Input: dimensioned drawing with shaded views. Units: mm. Origin: part minimum x, y, z. A direction names the side the tool comes from. Give positions to 0.01 mm unless a question says otherwise; leave off trailing zeros. Loops run counter-clockwise (first coordinate to the right, second up) from the corner with the lowest first, then second, coordinate; pieces in that order, holes last. Notation, with made-up numbers: (3.25, -5) -> (9.25, -5) arc R6 ccw to (9.25, 5) -> close; hole circle Ø11 at (65.25, 51). An arc over 180 degrees is marked (long way). One line per question, with ' | ' between items. Start each with the question number.
Item 1: Set-up query: the marked faces 4, 5, 6 and 7. Return all of +Z, -Z, +X, -X, +Y, -Y with unobstructed straight access to the full face (end or side cutting, diameter ignored); none if empty.
Item 2: Pin query (flat end, axial travel): P1, Ø1.9, axis at y = 2, z = 13, coming from the +X side; P2, Ø3, axis at x = 18.5, y = 3.5, coming from the -Z side; P3, Ø1.9, axis at y = 3.5, z = 4, coming from the +X side. Return the tip coordinate at first contact, or that it passes through.
Item 3: Section C-C on z = 24. Return loops of the section in (x, y), then the cut area to 3 significant figures.
Item 4: Section B-B on x = 27.5. Return loops of the section in (y, z).
Item 5: Material intervals for line 1 along X through (y, z) = (2.25, 6); line 2 along X through (y, z) = (1.5, 28.5); line 3 along Z through (x, y) = (10.5, 3.5), sorted ascending. Write a range as [from, to].
Item 6: Mould query, pull axis X, two halves, no side actions, for the marked faces 1, 2 and 3. Classes: released by +X, released by -X, zero draft, split by the parting line, or undercut.
Item 7: Section A-A on y = 4.25. Return loops of the section in (x, z) (3 decimals).
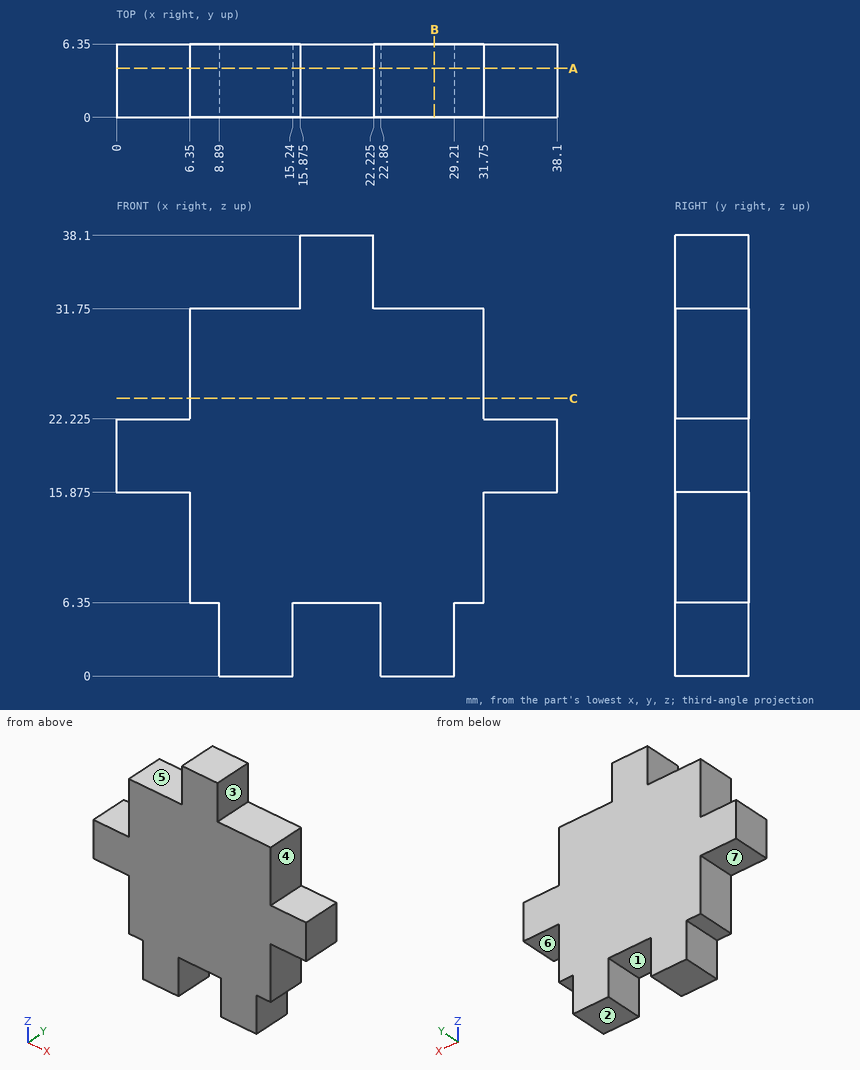
Result sheet:
1) face 4: +Z, +X, +Y, -Y | face 5: +Z, -X, +Y, -Y | face 6: -Z, +X, +Y, -Y | face 7: -Z, -X, +Y, -Y
2) P1: stops at x = 31.75 | P2: stops at z = 6.35 | P3: stops at x = 29.21
3) outline: (6.35, 0) -> (31.75, 0) -> (31.75, 6.35) -> (6.35, 6.35) -> close | area: 161 mm²
4) outline: (0, 0) -> (6.35, 0) -> (6.35, 31.75) -> (0, 31.75) -> close
5) line 1: x = [8.89, 15.24], [22.86, 29.21] | line 2: x = [6.35, 31.75] | line 3: z = [0, 31.75]
6) face 1: undercut | face 2: zero draft | face 3: released by +X
7) outline: (0, 15.875) -> (6.35, 15.875) -> (6.35, 6.35) -> (8.89, 6.35) -> (8.89, 0) -> (15.24, 0) -> (15.24, 6.35) -> (22.86, 6.35) -> (22.86, 0) -> (29.21, 0) -> (29.21, 6.35) -> (31.75, 6.35) -> (31.75, 15.875) -> (38.1, 15.875) -> (38.1, 22.225) -> (31.75, 22.225) -> (31.75, 31.75) -> (22.225, 31.75) -> (22.225, 38.1) -> (15.875, 38.1) -> (15.875, 31.75) -> (6.35, 31.75) -> (6.35, 22.225) -> (0, 22.225) -> close
